The listing builds one solid part. Answer for the finished solid, in the listing's coordinates (mm). Face numbers are marked on the shaded views. A direction names the side the tool comes from. Round coordinates to 2 decimals unless told otherwise and drop trailing zeros. Write each loop counter-clockwise with the first axis right and the second up, starting at its lowest first coordinate (ties: lowest second). Pieces come first, ordered by that corner, then holes.
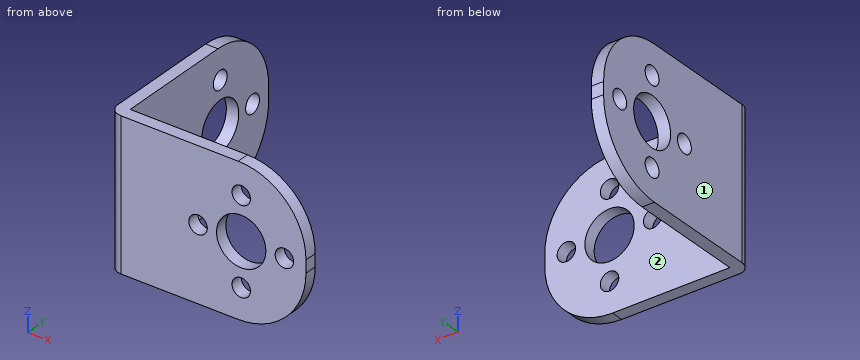
Autodesk Inventor part; units mm, degrees
ref_plane "YZ Plane" through (0, 0, 0) normal (1, 0, 0) x (0, 1, 0)
ref_plane "XZ Plane" through (0, 0, 0) normal (0, 1, 0) x (-1, 0, 0)
ref_plane "XY Plane" through (0, 0, 0) normal (0, 0, 1) x (1, 0, 0)
sketch "Эскиз1" plane through (0, 0, 0) normal (0, 1, 0) x (-1, 0, 0)
  line L0 (15.0734, 10.2239) -> (-16.9266, 10.2239)
  line L1 (-16.9266, 10.2239) -> (-16.9266, -13.7761)
  line L2 (-16.9266, -13.7761) -> (15.0734, -13.7761)
  line L3 (15.0734, -13.7761) -> (15.0734, 10.2239)
  point P0 (0, 0)
  dimension "d0" = 32
  dimension "d1" = 24
extrude "Выдавливание1" add sketch "Эскиз1" along normal blind 2
sketch "Эскиз2" plane through (0, 2, 0) normal (0, 1, 0) x (1, 0, 0)
  line L0 (16.9266, 13.7761) -> (-15.0734, 13.7761)
  line L1 (-15.0734, -10.2239) -> (16.9266, -10.2239)
  line L2 (-15.0734, 13.7761) -> (-13.0734, 13.7761)
  line L3 (-13.0734, 13.7761) -> (-13.0734, -10.2239)
  line L4 (-13.0734, -10.2239) -> (-15.0734, -10.2239)
  line L5 (-15.0734, -10.2239) -> (-15.0734, 13.7761)
  point P0 (0, 0)
  dimension "d4" = 2
extrude "Выдавливание2" add sketch "Эскиз2" along normal blind 30
sketch "Эскиз3" plane through (-13.0734, 2, 10.2239) normal (1, 0, 0) x (0, 0, -1)
  circle A0 centre (12, 19.5) radius 4
  circle A1 centre (12, 19.5) radius 7
  line L0 (24, 30) -> (0, 30)
  line L1 (24, 0) -> (24, 30)
  circle A2 centre (19, 19.5) radius 1.5
  circle A3 centre (12, 12.5) radius 1.5
  circle A4 centre (5, 19.5) radius 1.5
  circle A5 centre (12, 26.5) radius 1.5
  point P0 (10.2239, -2)
  point P1 (12, 30)
  dimension "d7" = 8
  dimension "d8" = 14
  dimension "d10" = 12
  dimension "d11" = 3
  dimension "d12" = 3
  dimension "d13" = 3
  dimension "d14" = 3
  dimension "d15" = 3.5
  dimension "d16" = 0
  dimension "d17" = 0
  dimension "d18" = 0
  dimension "d19" = 7
extrude "Выдавливание3" cut sketch "Эскиз3" against normal blind 100 contours A0 | A1 A2 | A1 A2 | A5 A1 | A1 A5 | A3 A1 | A1 A3 | A4 A1 | A1 A4
sketch "Эскиз4" plane through (0, 2, 0) normal (0, 1, 0) x (1, 0, 0)
  circle A0 centre (6.4266, 1.7761) radius 4
  circle A1 centre (6.4266, 1.7761) radius 7
  circle A2 centre (6.4266, -5.2239) radius 1.5
  circle A3 centre (6.4266, 8.7761) radius 1.5
  circle A4 centre (-0.5734, 1.7761) radius 1.5
  circle A5 centre (13.4266, 1.7761) radius 1.5
  line L0 (16.9266, -10.2239) -> (16.9266, 13.7761)
  line L1 (16.9266, 13.7761) -> (-13.0734, 13.7761)
  point P0 (0, 0)
  point P1 (16.9266, 1.7761)
  dimension "d22" = 8
  dimension "d23" = 14
  dimension "d24" = 3
  dimension "d25" = 3
  dimension "d26" = 3
  dimension "d27" = 3
  dimension "d29" = 12
  dimension "d30" = 3.5
extrude "Выдавливание4" cut sketch "Эскиз4" against normal blind 100 contours A0 | A1 A5 | A1 A5 | A3 A1 | A1 A3 | A2 A1 | A1 A2 | A4 A1 | A1 A4
fillet "Сопряжение1" radius 11 4 edges at (-14.0734, 32, 10.2239) (-14.0734, 32, -13.7761) (16.9266, 1, -13.7761) (16.9266, 1, 10.2239)
fillet "Сопряжение2" radius 2 1 edges at (-15.0734, 0, -1.7761)
properties part number "уголок" material "Сталь"
1. Straight lines are drawn through the part: line 1 along Y through (x, z) = (10.5, 8.25); line 2 along X through (y, z) = (4, -6); line 3 along Y through (x, z) = (-14, -4.5). For each, find the intervals that lie inside material, in ascending order.
Geometry says:
line 1: y = 0 to 2
line 2: x = -15.07 to -13.07
line 3: y = 0.23 to 18.57, 24.43 to 31.86
2. Section B-B on x = 3 is taken. Determine the outline of the cut face in (y, z), plus the area to 3 significant figures.
Geometry says:
outline: (0, -13.78) - (2, -13.78) - (2, -3.84) - (0, -3.84) - close; (0, 0.29) - (2, 0.29) - (2, 10.22) - (0, 10.22) - close
area: 39.7 mm2
3. Section C-C on y = 21.5 is taken. Determine the outline of the cut face in (x, z), plus the area to 3 significant figures.
Geometry says:
outline: (-15.07, -13.76) - (-13.07, -13.76) - (-13.07, -10.28) - (-15.07, -10.28) - close; (-15.07, -7.28) - (-13.07, -7.28) - (-13.07, -5.78) - (-15.07, -5.78) - close; (-15.07, 2.22) - (-13.07, 2.22) - (-13.07, 3.72) - (-15.07, 3.72) - close; (-15.07, 6.72) - (-13.07, 6.72) - (-13.07, 10.21) - (-15.07, 10.21) - close
area: 20.0 mm2
4. Section D-D on z = 3 is taken. Determine the outline of the cut face in (x, y).
Geometry says:
outline: (-15.07, 2) arc R2 ccw to (-13.07, 0) - (16.26, 0) - (16.26, 2) - (-13.07, 2) - (-13.07, 31.33) - (-15.07, 31.33) - close
5. Section A-A on y = 14.5 is taken. Determine the outline of the cut face in (x, z), plus the area to 3 significant figures.
Geometry says:
outline: (-15.07, -13.78) - (-13.07, -13.78) - (-13.07, -3.28) - (-15.07, -3.28) - close; (-15.07, -0.28) - (-13.07, -0.28) - (-13.07, 10.22) - (-15.07, 10.22) - close
area: 42.0 mm2
6. Given pin 1 (1.5 mm diameter, centred on x = 12.5, y = 4, fed in from +Z); pin 2 (10.5 mm diameter, centred on x = 6.43, z = -1.78, fed in from +Y); pin 3 (1 mm diameter, centred on y = 10.5, z = -8, fed in from +X), each flat-ended and moving along its own axis, determine where each tip first touches the part or whether it passes through.
Geometry says:
pin 1: passes through
pin 2: stops at y = 2
pin 3: stops at x = -13.07
7. A tool of negligible diameter and unlimited length cuts with its end or side. For the marked faces 1 and 2, from which of +Z, -Z, +X, -X, +Y, -Y can it reach the whole face along a straight path? Write none if from no direction.
Geometry says:
face 1: +Z, -Z, -X, +Y, -Y
face 2: +Z, -Z, +X, +Y
